Could you check a few things on this model? Use its own coordinates, in mm. Give positions to 0.01 mm unless a question says otherwise; leave off trailing zeros. Write each loop counter-clockwise with the first axis right and the second up, starting at its lowest first coordinate (ties: lowest second). Pieces come first, ordered by that corner, then holes. Notation, with made-up numbers: (4.25, 74) - (18.25, 74) arc R20 cw to (18.25, 109) - close; hole circle Ø7 at (15, 40). An arc over 180 degrees is marked (long way). Answer as a JSON object with one key per item and string values. Group by question number.
```python
from build123d import *

# Parameters (mm, degrees)
F0_W     = 1016
F0_H     = 355.6
F1_DEPTH = 19.05
F3_DEPTH = 19.051
F5_DEPTH = 19.051
F6_W     = 6.35
F6_H     = 152.4
F7_DEPTH = 19.051


with BuildPart() as f1:
    # F0 (on Top) → F1 (new body)
    with BuildSketch(Plane.XY):
        with Locations((-22.724911, -38.823086)):
            Rectangle(F0_W, F0_H)
    extrude(amount=F1_DEPTH)

    # F2 (on face) → F3 (cut, through all)
    with BuildSketch(Plane.XY.offset(19.05)):
        with BuildLine():
            Line((-403.724911, 138.976914), (-441.824911, 138.976914))
            Line((-441.824911, 138.976914), (-441.824911, 94.526914))
            ThreePointArc((-441.824911, 94.526914), (-422.774911, 75.476914), (-403.724911, 94.526914))
            Line((-403.724911, 94.526914), (-403.724911, 138.976914))
        make_face()
        with BuildLine():
            Line((-441.824911, -216.623086), (-441.824911, -172.173086))
            ThreePointArc((-441.824911, -172.173086), (-460.874911, -153.123086), (-479.924911, -172.173086))
            Line((-479.924911, -172.173086), (-479.924911, -216.623086))
            Line((-479.924911, -216.623086), (-441.824911, -216.623086))
        make_face()
        with BuildLine():
            Line((-327.524911, 138.976914), (-365.624911, 138.976914))
            Line((-365.624911, 138.976914), (-365.624911, 94.526914))
            ThreePointArc((-365.624911, 94.526914), (-346.574911, 75.476914), (-327.524911, 94.526914))
            Line((-327.524911, 94.526914), (-327.524911, 138.976914))
        make_face()
        with BuildLine():
            Line((-365.624911, -216.623086), (-365.624911, -172.173086))
            ThreePointArc((-365.624911, -172.173086), (-384.674911, -153.123086), (-403.724911, -172.173086))
            Line((-403.724911, -172.173086), (-403.724911, -216.623086))
            Line((-403.724911, -216.623086), (-365.624911, -216.623086))
        make_face()
        with BuildLine():
            Line((-251.324911, 138.976914), (-289.424911, 138.976914))
            Line((-289.424911, 138.976914), (-289.424911, 94.526914))
            ThreePointArc((-289.424911, 94.526914), (-270.374911, 75.476914), (-251.324911, 94.526914))
            Line((-251.324911, 94.526914), (-251.324911, 138.976914))
        make_face()
        with BuildLine():
            Line((-289.424911, -216.623086), (-289.424911, -172.173086))
            ThreePointArc((-289.424911, -172.173086), (-308.474911, -153.123086), (-327.524911, -172.173086))
            Line((-327.524911, -172.173086), (-327.524911, -216.623086))
            Line((-327.524911, -216.623086), (-289.424911, -216.623086))
        make_face()
        with BuildLine():
            Line((-175.124911, 138.976914), (-213.224911, 138.976914))
            Line((-213.224911, 138.976914), (-213.224911, 94.526914))
            ThreePointArc((-213.224911, 94.526914), (-194.174911, 75.476914), (-175.124911, 94.526914))
            Line((-175.124911, 94.526914), (-175.124911, 138.976914))
        make_face()
        with BuildLine():
            Line((-213.224911, -216.623086), (-213.224911, -172.173086))
            ThreePointArc((-213.224911, -172.173086), (-232.274911, -153.123086), (-251.324911, -172.173086))
            Line((-251.324911, -172.173086), (-251.324911, -216.623086))
            Line((-251.324911, -216.623086), (-213.224911, -216.623086))
        make_face()
        with BuildLine():
            Line((-98.924911, 138.976914), (-137.024911, 138.976914))
            Line((-137.024911, 138.976914), (-137.024911, 94.526914))
            ThreePointArc((-137.024911, 94.526914), (-117.974911, 75.476914), (-98.924911, 94.526914))
            Line((-98.924911, 94.526914), (-98.924911, 138.976914))
        make_face()
        with BuildLine():
            Line((-137.024911, -216.623086), (-137.024911, -172.173086))
            ThreePointArc((-137.024911, -172.173086), (-156.074911, -153.123086), (-175.124911, -172.173086))
            Line((-175.124911, -172.173086), (-175.124911, -216.623086))
            Line((-175.124911, -216.623086), (-137.024911, -216.623086))
        make_face()
        with BuildLine():
            Line((-22.724911, 138.976914), (-60.824911, 138.976914))
            Line((-60.824911, 138.976914), (-60.824911, 94.526914))
            ThreePointArc((-60.824911, 94.526914), (-41.774911, 75.476914), (-22.724911, 94.526914))
            Line((-22.724911, 94.526914), (-22.724911, 138.976914))
        make_face()
        with BuildLine():
            Line((-60.824911, -216.623086), (-60.824911, -172.173086))
            ThreePointArc((-60.824911, -172.173086), (-79.874911, -153.123086), (-98.924911, -172.173086))
            Line((-98.924911, -172.173086), (-98.924911, -216.623086))
            Line((-98.924911, -216.623086), (-60.824911, -216.623086))
        make_face()
        with BuildLine():
            Line((53.475089, 138.976914), (15.375089, 138.976914))
            Line((15.375089, 138.976914), (15.375089, 94.526914))
            ThreePointArc((15.375089, 94.526914), (34.425089, 75.476914), (53.475089, 94.526914))
            Line((53.475089, 94.526914), (53.475089, 138.976914))
        make_face()
        with BuildLine():
            Line((15.375089, -216.623086), (15.375089, -172.173086))
            ThreePointArc((15.375089, -172.173086), (-3.674911, -153.123086), (-22.724911, -172.173086))
            Line((-22.724911, -172.173086), (-22.724911, -216.623086))
            Line((-22.724911, -216.623086), (15.375089, -216.623086))
        make_face()
        with BuildLine():
            Line((129.675089, 138.976914), (91.575089, 138.976914))
            Line((91.575089, 138.976914), (91.575089, 94.526914))
            ThreePointArc((91.575089, 94.526914), (110.625089, 75.476914), (129.675089, 94.526914))
            Line((129.675089, 94.526914), (129.675089, 138.976914))
        make_face()
        with BuildLine():
            Line((91.575089, -216.623086), (91.575089, -172.173086))
            ThreePointArc((91.575089, -172.173086), (72.525089, -153.123086), (53.475089, -172.173086))
            Line((53.475089, -172.173086), (53.475089, -216.623086))
            Line((53.475089, -216.623086), (91.575089, -216.623086))
        make_face()
        with BuildLine():
            Line((205.875089, 138.976914), (167.775089, 138.976914))
            Line((167.775089, 138.976914), (167.775089, 94.526914))
            ThreePointArc((167.775089, 94.526914), (186.825089, 75.476914), (205.875089, 94.526914))
            Line((205.875089, 94.526914), (205.875089, 138.976914))
        make_face()
        with BuildLine():
            Line((167.775089, -216.623086), (167.775089, -172.173086))
            ThreePointArc((167.775089, -172.173086), (148.725089, -153.123086), (129.675089, -172.173086))
            Line((129.675089, -172.173086), (129.675089, -216.623086))
            Line((129.675089, -216.623086), (167.775089, -216.623086))
        make_face()
        with BuildLine():
            Line((282.075089, 94.526914), (282.075089, 138.976914))
            Line((282.075089, 138.976914), (243.975089, 138.976914))
            Line((243.975089, 138.976914), (243.975089, 94.526914))
            ThreePointArc((243.975089, 94.526914), (263.025089, 75.476914), (282.075089, 94.526914))
        make_face()
        with BuildLine():
            Line((243.975089, -216.623086), (243.975089, -172.173086))
            ThreePointArc((243.975089, -172.173086), (224.925089, -153.123086), (205.875089, -172.173086))
            Line((205.875089, -172.173086), (205.875089, -216.623086))
            Line((205.875089, -216.623086), (243.975089, -216.623086))
        make_face()
        with BuildLine():
            Line((358.275089, 94.526914), (358.275089, 138.976914))
            Line((358.275089, 138.976914), (320.175089, 138.976914))
            Line((320.175089, 138.976914), (320.175089, 94.526914))
            ThreePointArc((320.175089, 94.526914), (339.225089, 75.476914), (358.275089, 94.526914))
        make_face()
        with BuildLine():
            Line((320.175089, -216.623086), (320.175089, -172.173086))
            ThreePointArc((320.175089, -172.173086), (301.125089, -153.123086), (282.075089, -172.173086))
            Line((282.075089, -172.173086), (282.075089, -216.623086))
            Line((282.075089, -216.623086), (320.175089, -216.623086))
        make_face()
        with BuildLine():
            Line((434.475089, 94.526914), (434.475089, 138.976914))
            Line((434.475089, 138.976914), (396.375089, 138.976914))
            Line((396.375089, 138.976914), (396.375089, 94.526914))
            ThreePointArc((396.375089, 94.526914), (415.425089, 75.476914), (434.475089, 94.526914))
        make_face()
        with BuildLine():
            Line((396.375089, -216.623086), (396.375089, -172.173086))
            ThreePointArc((396.375089, -172.173086), (377.325089, -153.123086), (358.275089, -172.173086))
            Line((358.275089, -172.173086), (358.275089, -216.623086))
            Line((358.275089, -216.623086), (396.375089, -216.623086))
        make_face()
    extrude(amount=-F3_DEPTH, mode=Mode.SUBTRACT)

    # F4 (on face) → F5 (cut, through all)
    with BuildSketch(Plane.XY.offset(19.05)):
        Polygon((-518.024911, -115.023086), (-518.024911, -38.823086), (-518.024911, 37.376914), (-530.724911, 37.376914), (-530.724911, -38.823086), (-530.724911, -115.023086), align=None)
        Polygon((485.275089, 37.376914), (472.575089, 37.376914), (472.575089, -38.823086), (472.575089, -115.023086), (485.275089, -115.023086), (485.275089, -38.823086), align=None)
    extrude(amount=-F5_DEPTH, mode=Mode.SUBTRACT)

    # F6 (on face) → F7 (cut, through all)
    with BuildSketch(Plane.XY.offset(19.05)):
        with Locations((-514.849911, -38.823086)):
            Rectangle(F6_W, F6_H)
        with Locations((469.400089, -38.823086)):
            Rectangle(F6_W, F6_H)
    extrude(amount=-F7_DEPTH, mode=Mode.SUBTRACT)


solid = f1.part
```
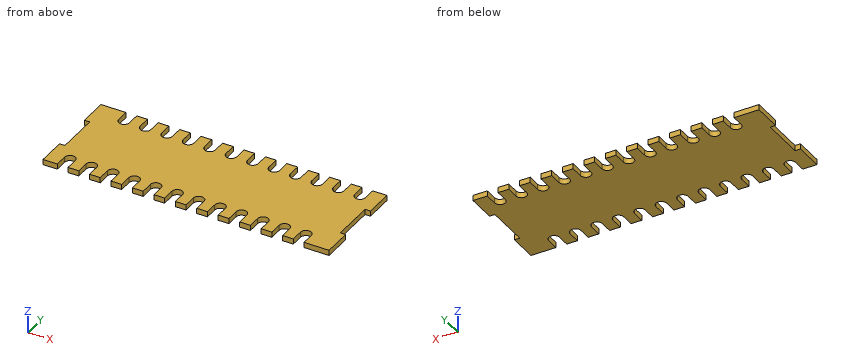
(1) I want a section at B-B, the plane y = -71. Please give me the cut outline in (x, z).
(2) I want a section at C-C, the plane x = 406.5. Please give me the cut outline in (y, z).
(3) Will these pins go through, and if not, where does the flat tip stop? P1, Ø5, axis at y = -101, z = 3, coming from the +X side; P2, Ø10, axis at x = -161, z = 2, coming from the -Y side; P3, Ø1, axis at x = -64, z = 6, coming from the -Y side.
(4) I want a section at A-A, the plane y = 104.5. State how many separate pieces and enclosed holes the cut face has, and give its area (3 significant figures).
(5) I need wall thicknesses on L1, parallel to X at y = 14.5, z = 16; L2, parallel to Y at x = 416, z = 8.5; L3, parallel to Y at x = 402.5, z = 1.5. Which ranges of each line are inside material? Lowest first, please.
Entries:
{
 "1": {"outline": "(-511.67, 0) - (466.23, 0) - (466.23, 19.05) - (-511.67, 19.05) - close"},
 "2": {"outline": "(-216.62, 0) - (77.7, 0) - (77.7, 19.05) - (-216.62, 19.05) - close"},
 "3": {"P1": "x = 466.23", "P2": "y = -155.91", "P3": "y = -162.44"},
 "4": {"separate pieces": "13", "enclosed holes": "0", "area": "10,600 mm^2"},
 "5": {"L1": "-511.67 to 466.23", "L2": "-216.62 to 75.49", "L3": "-216.62 to 80.53"}
}
